Autodesk Inventor part; units mm, degrees
ref_plane "YZ Plane" through (0, 0, 0) normal (1, 0, 0) x (0, 1, 0)
ref_plane "XZ Plane" through (0, 0, 0) normal (0, 1, 0) x (-1, 0, 0)
ref_plane "XY Plane" through (0, 0, 0) normal (0, 0, 1) x (1, 0, 0)
sketch "Sketch1" plane through (0, 0, 0) normal (0, 0, 1) x (1, 0, 0)
  line L0 (139.7, -3.175) -> (-139.7, -3.175)
  line L1 (-139.7, -3.175) -> (-139.7, 3.175)
  line L2 (-139.7, 3.175) -> (139.7, 3.175)
  line L3 (139.7, 3.175) -> (139.7, -3.175)
  line L4 (139.7, -3.175) -> (-139.7, 3.175) construction
  line L5 (-139.7, -3.175) -> (139.7, 3.175) construction
  point P0 (0, 0)
  dimension "d0" = 279.4
  dimension "d1" = 6.35
extrude "Extrusion1" add sketch "Sketch1" along normal blind 63.5
sketch "Sketch2" plane through (-139.7, 3.175, 0) normal (0, 1, 0) x (1, 0, 0)
  circle A0 centre (140.335, -26) radius 4.445
  line L0 (139.7, 0) -> (139.7, -63.5833) construction
  line L1 (0, 0) -> (0, -63.5) construction
  line L2 (279.4, 0) -> (279.4, -63.5) construction
  line L3 (279.4, -63.5) -> (0, -63.5)
  dimension "d4" = 8.89
  dimension "d16" = 37.5
extrude "Extrusion2" cut sketch "Sketch2" against normal through all
sketch "Sketch3" plane through (0, 0, 63.5) normal (0, 0, 1) x (1, 0, 0)
  point P0 (0, 0)
sketch "Sketch4" plane through (-139.7, 3.175, 0) normal (0, 1, 0) x (1, 0, 0)
  line L0 (279.4, 0) -> (279.4, -63.5)
  line L1 (0, 0) -> (0, -63.5)
  line L2 (279.4, -63.5) -> (0, -63.5)
  line L3 (0, -63.5) -> (0, -57.15)
  line L4 (0, -57.15) -> (279.4, -57.15)
  line L5 (279.4, -57.15) -> (279.4, -63.5)
  point P0 (139.7, 0)
  dimension "d8" = 6.35
extrude "Extrusion3" add sketch "Sketch4" along normal blind 63.5
sketch "Sketch5" plane through (0, 0, 63.5) normal (0, 0, 1) x (1, 0, 0)
  line L0 (47.5, 14.825) -> (-47.5, 14.825)
  line L1 (-47.5, 14.825) -> (-47.5, 45.305)
  line L2 (-47.5, 45.305) -> (47.5, 45.305)
  line L3 (47.5, 45.305) -> (47.5, 14.825)
  line L4 (47.5, 14.825) -> (-47.5, 45.305) construction
  line L5 (-47.5, 14.825) -> (47.5, 45.305) construction
  line L6 (-139.7, -3.175) -> (139.7, -3.175)
  point P0 (0, 0)
  point P1 (0, 30.065)
  dimension "d11" = 95
  dimension "d12" = 30.48
  dimension "d13" = 18
extrude "Extrusion4" cut sketch "Sketch5" against normal through all
sketch "Sketch8" plane through (0, 0, 63.5) normal (0, 0, 1) x (1, 0, 0)
  line L0 (-139.7, -3.175) -> (139.7, -3.175) construction
  line L1 (-47.5, -3.175) -> (-47.5, 66.9222) construction
  line L2 (-139.7, 66.675) -> (139.7, 66.675) construction
  line L3 (47.5, 66.675) -> (47.5, -3.175) construction
  line L4 (47.5, 45.305) -> (47.5, 14.825) construction
  line L5 (-47.5, 14.825) -> (-47.5, 45.305) construction
  line L6 (-139.7, -3.175) -> (-139.7, 66.675) construction
  line L7 (-139.7, 3.175) -> (139.7, 3.175) construction
  line L8 (139.7, -3.175) -> (139.7, 66.675) construction
  line L9 (-139.7, 55.753) -> (139.7, 55.753)
  line L10 (-47.5, 55.753) -> (-139.7, 3.175)
  line L11 (47.5, 55.753) -> (139.7, 3.175)
  line L12 (-47.5, 14.825) -> (-47.5, 45.305)
  line L13 (-47.5, 45.305) -> (47.5, 45.305)
  line L14 (47.5, 45.305) -> (47.5, 14.825)
  line L15 (47.5, 14.825) -> (-47.5, 14.825)
  line L16 (-139.7, -3.175) -> (-139.7, 66.675)
  line L17 (-139.7, -3.175) -> (139.7, -3.175)
  line L18 (139.7, -3.175) -> (139.7, 66.675)
  line L19 (-139.7, 66.675) -> (139.7, 66.675)
  point P0 (0, 0)
  point P1 (-47.5, 30.065)
  point P2 (-139.7, 3.175)
  point P3 (139.7, 3.175)
  dimension "d21" = 0
  dimension "d22" = 0
  dimension "d23" = 6.35
  dimension "d24" = 10.922
extrude "Extrusion5" cut sketch "Sketch8" against normal through all contours L16 L19 L18 L9 | L9 L10 L16 | L9 L18 L11
sketch "Sketch11" plane through (-139.7, 3.175, 0) normal (0, 1, 0) x (1, 0, 0)
  circle A0 centre (140.335, -26) radius 4.445
  circle A1 centre (140.335, -26) radius 12.7
  line L0 (127.635, -26) -> (0, -26)
  line L1 (0, 0) -> (0, -57.15)
  line L2 (153.035, -26) -> (279.4, -26)
  line L3 (279.4, 0) -> (279.4, -57.15)
  line L4 (279.4, 0) -> (0, 0)
  point P0 (139.7, 0)
  point P1 (0, -34.9602)
  point P2 (280.67, -34.9602)
  point P3 (279.4, -57.15)
  dimension "d43" = 25.4
extrude "Extrusion8" cut sketch "Sketch11" against normal through all contours A1 L0 L1 L4 L3 L2
fillet "Fillet5" radius 6.35 6 edges at (47.5, 55.753, 60.325) (-47.5, 55.753, 60.325) (139.7, 0, 26) (13.335, 0, 26) (-12.065, 0, 26) (-139.7, 0, 26)
sketch "Sketch15" plane through (-139.7, -3.175, 63.5) normal (-1, 0, 0) x (0, 0, 1)
  circle A0 centre (-4, -5) radius 2.5
  line L0 (-31.15, 0) -> (-31.15, 6.35)
  line L1 (-31.15, 0) -> (0, 0)
  line L2 (0, 0) -> (0, 6.35)
  line L3 (0, 6.35) -> (-6.35, 6.35)
  line L4 (-31.15, 6.35) -> (-6.35, 6.35)
  line L5 (0, 0) -> (0, -21.002)
  circle A1 centre (-4, -21.002) radius 2.5
  circle A2 centre (-4, -21.002) radius 4
  line L6 (-31.15, 0) -> (0, 0)
  line L7 (-31.15, 0) -> (-6.7994, -23.8591)
  point P0 (-63.5, 3.175)
  dimension "d64" = 5
  dimension "d65" = 4
  dimension "d66" = 5
  dimension "d67" = 5
  dimension "d68" = 16.002
extrude "Extrusion11" add sketch "Sketch15" against normal blind 6.35 contours L1 L5 A2 L7 | A2
sketch "Sketch16" plane through (139.7, -3.175, 63.5) normal (1, 0, 0) x (0, 0, -1)
  line L0 (0, 0) -> (0, -21.002)
  arc A0 (0, -21.002) -> (6.7994, -23.8591) centre (4, -21.002) ccw
  line L1 (6.7994, -23.8591) -> (31.15, 0)
  line L2 (0, 0) -> (31.15, 0)
  circle A1 centre (4, -5) radius 2.5
  circle A2 centre (4, -21.002) radius 2.5
  point P0 (63.5, 3.175)
extrude "Extrusion12" add sketch "Sketch16" against normal blind 6.35
properties part number "CS_Camera_Mount"
Part model, mm, in its own coordinate system. A direction names the side the tool comes from. Round coordinates to 2 decimals unless told otherwise and drop trailing zeros. Write each loop counter-clockwise with the first axis right and the second up, starting at its lowest first coordinate (ties: lowest second). Pieces come first, ordered by that corner, then holes. Notation, with made-up numbers: M 14,-16 L 72,-16 A9 ccw 72,-5 Z; hole C 37,-15.5 d6. An arc over 180 degrees is marked long. Answer as CSV lines item,"result". Start each with the question number.
1) Which spindle directions (+Z, -Z, +X, -X, +Y, -Y) get a long thin tool onto all of the face, cutting with end or side? Do faces 1 (the face through (137.79, -0.04, 27.81)), 2 (the face through (-2, 12, 57.15)), 3 (the face through (47.5, 30, 60)), 4 (the face through (133.35, -13, 52)), 5 (the face through (-136.569, -22.069, 60.844)). Say none if no direction does.
2) Band-saw the part on A-A (y = 28). List the corners of the cut face in (x, z), then the cut area to 3 significant figures.
3) Band-saw the part on D-D (x = 53.5). List the corners of the cut face in (y, z) (3 decimals), then the cut area to 3 significant figures.
4) Band-saw the part on C-C (z = 52). List the corners of the cut face in (x, y) (3 decimals), then the cut area to 3 significant figures.
5) Drill centre lines: L1, parallel to X at y = -6, z = 41; L2, parallel to Y at x = -135.25, z = 59.5 (3 decimals); L3, parallel to Z at x = 36, y = 8.5. Where is each one in solid material? Low to high.
6) Drop flat-ended pins along their axis: pin 1 (1.5 mm diameter, centred on x = -53.5, z = 49.5, fed in from +Y) (3 decimals); pin 2 (5 mm diameter, centred on x = -96.5, y = 0.5, fed in from -Z); pin 3 (7 mm diameter, centred on y = 30, z = 61, fed in from -X). Give the stop position or say it passes through.
7) Mould opens along X. For faces 6 (the face through (0.056, 0.044, 21.593)), 7 (the face through (-137.89, -0.04, 27.91)), 8 (the face through (-136.569, -14.938, 44.355)) say: +X half, -X half, draft (parallel to the pull), parting line (faces both ways), or undercut.
8) Band-saw the part on B-B (x = -122). List the corners of the cut face in (y, z) (3 decimals), then the cut area to 3 significant figures.
Worked out:
1,face 1,"-Z, +X, +Y, -Y"
1,face 2,"-Z, +X, -X, +Y"
1,face 3,"+Z, -Z"
1,face 4,"+Z, -Z, -Y"
1,face 5,"+X, -X"
2,outline,"M -96.17,57.15 L -47.5,57.15 L -47.5,63.5 L -96.17,63.5 Z; M 47.5,57.15 L 96.17,57.15 L 96.17,63.5 L 47.5,63.5 Z"
2,area,"618 mm²"
3,outline,"M -3.175,26 L 3.175,26 L 3.175,57.15 L 52.331,57.15 L 52.331,63.5 L -3.175,63.5 Z"
3,area,"550 mm²"
4,outline,"M -139.7,-22.428 L -133.35,-22.428 L -133.35,-3.175 L 133.35,-3.175 L 133.35,-22.428 L 139.7,-22.428 L 139.7,3.175 L -139.7,3.175 Z"
4,area,"2,020 mm²"
5,L1,"-139.7 to -133.35, 133.35 to 139.7"
5,L2,"-28.177 to -26.677, -21.677 to -10.675, -5.675 to 5.713"
5,L3,"57.15 to 63.5"
6,pin 1,"y = 3.175"
6,pin 2,"z = 26"
6,pin 3,"x = -98.8"
7,face 6,"undercut"
7,face 7,"-X half"
7,face 8,"draft"
8,outline,"M -3.175,26 L 3.175,26 L 3.175,57.15 L 13.269,57.15 L 13.269,63.5 L -3.175,63.5 Z"
8,area,"302 mm²"
